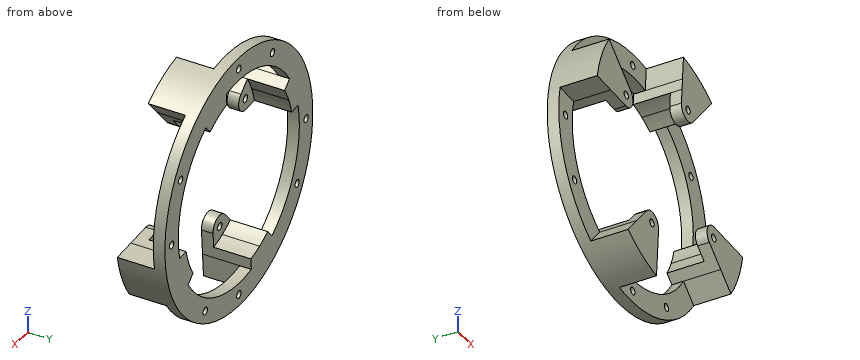
from build123d import *

# Parameters (mm, degrees)
SKETCH1_R           = 55
SKETCH1_R_2         = 1.6
BOSS_EXTRUDE8_DEPTH = 21
CUT_EXTRUDE1_DEPTH  = 16
CUT_EXTRUDE7_START  = 21
SKETCH1_22_R        = 5
SKETCH1_22_R_2      = 1.6
CUT_EXTRUDE7_DEPTH  = 16
SKETCH6_R           = 1.6
CUT_EXTRUDE8_DEPTH  = 81.566742518


with BuildPart() as part:
    # Sketch1 → Boss-Extrude8 (new body)
    with BuildSketch(Plane(origin=(0, 0, 0), x_dir=(1, 0, 0), z_dir=(0, 1, 0))):
        with Locations(Location((0, 0, 0), (0, 0, 90))):
            Circle(SKETCH1_R)
        with BuildLine():
            Line((-24.560877041, 37.706276918), (-17.257446053, 29.262481604))
            ThreePointArc((-17.257446053, 29.262481604), (-11.562365731, 27.91402016), (-8.488842047, 32.894556307))
            Line((-8.488842047, 32.894556307), (-9.295201395, 44.029526809))
            ThreePointArc((-9.295201395, 44.029526809), (17.220754456, 41.574578963), (37.706276918, 24.560877041))
            Line((37.706276918, 24.560877041), (29.262481604, 17.257446053))
            ThreePointArc((29.262481604, 17.257446053), (27.91402016, 11.562365731), (32.894556307, 8.488842047))
            Line((32.894556307, 8.488842047), (44.029526809, 9.295201395))
            ThreePointArc((44.029526809, 9.295201395), (41.574578963, -17.220754456), (24.560877041, -37.706276918))
            Line((24.560877041, -37.706276918), (17.257446053, -29.262481604))
            ThreePointArc((17.257446053, -29.262481604), (11.562365731, -27.91402016), (8.488842047, -32.894556307))
            Line((8.488842047, -32.894556307), (8.94591471, -39.206246783))
            Line((8.94591471, -39.206246783), (9.295201395, -44.029526809))
            ThreePointArc((9.295201395, -44.029526809), (-17.220754456, -41.574578963), (-37.706276918, -24.560877041))
            Line((-37.706276918, -24.560877041), (-34.04871992, -21.39728601))
            Line((-34.04871992, -21.39728601), (-29.262481604, -17.257446053))
            ThreePointArc((-29.262481604, -17.257446053), (-27.91402016, -11.562365731), (-32.894556307, -8.488842047))
            Line((-32.894556307, -8.488842047), (-44.029526809, -9.295201395))
            ThreePointArc((-44.029526809, -9.295201395), (-41.574578963, 17.220754456), (-24.560877041, 37.706276918))
        make_face(mode=Mode.SUBTRACT)
        with Locations(Location((-13.475782892, 32.533417823, 0), (0, 0, 90))):
            Circle(SKETCH1_R_2, mode=Mode.SUBTRACT)
        with Locations(Location((32.533417823, 13.475782892, 0), (0, 0, 90))):
            Circle(SKETCH1_R_2, mode=Mode.SUBTRACT)
        with Locations(Location((-32.533417823, -13.475782892, 0), (0, 0, 90))):
            Circle(SKETCH1_R_2, mode=Mode.SUBTRACT)
        with Locations(Location((13.475782892, -32.533417823, 0), (0, 0, 90))):
            Circle(SKETCH1_R_2, mode=Mode.SUBTRACT)
    extrude(amount=BOSS_EXTRUDE8_DEPTH)

    # Sketch1_15 → Cut-Extrude1 (cut)
    with BuildSketch(Plane(origin=(0, 0, 0), x_dir=(1, 0, 0), z_dir=(0, 1, 0))):
        with BuildLine():
            ThreePointArc((-9.295201395, 44.029526809), (17.220754456, 41.574578963), (37.706276918, 24.560877041))
            Line((37.706276918, 24.560877041), (45.326940374, 31.152343031))
            ThreePointArc((45.326940374, 31.152343031), (21.04758878, 50.813374288), (-10.022953902, 54.079019916))
            Line((-10.022953902, 54.079019916), (-9.295201395, 44.029526809))
        make_face()
        with BuildLine():
            ThreePointArc((-44.029526809, -9.295201395), (-41.574578963, 17.220754456), (-24.560877041, 37.706276918))
            Line((-24.560877041, 37.706276918), (-31.152343031, 45.326940374))
            ThreePointArc((-31.152343031, 45.326940374), (-50.813374288, 21.04758878), (-54.079019916, -10.022953902))
            Line((-54.079019916, -10.022953902), (-44.029526809, -9.295201395))
        make_face()
        with BuildLine():
            Line((54.079019916, 10.022953902), (44.029526809, 9.295201395))
            ThreePointArc((44.029526809, 9.295201395), (41.574578963, -17.220754456), (24.560877041, -37.706276918))
            Line((24.560877041, -37.706276918), (31.152343031, -45.326940374))
            ThreePointArc((31.152343031, -45.326940374), (50.813374288, -21.04758878), (54.079019916, 10.022953902))
        make_face()
        with BuildLine():
            ThreePointArc((9.295201395, -44.029526809), (-17.220754456, -41.574578963), (-37.706276918, -24.560877041))
            Line((-37.706276918, -24.560877041), (-45.326940374, -31.152343031))
            ThreePointArc((-45.326940374, -31.152343031), (-21.04758878, -50.813374288), (10.022953902, -54.079019916))
            Line((10.022953902, -54.079019916), (9.295201395, -44.029526809))
        make_face()
    extrude(amount=CUT_EXTRUDE1_DEPTH, mode=Mode.SUBTRACT)

    # Sketch1_22 → Cut-Extrude7 (cut)
    with BuildSketch(Plane(origin=(0, 0, 0), x_dir=(1, 0, 0), z_dir=(0, 1, 0)).offset(CUT_EXTRUDE7_START)):
        with Locations((13.475782892, -32.533417823)):
            Circle(SKETCH1_22_R)
        with Locations(Location((13.475782892, -32.533417823, 0), (0, 0, 90))):
            Circle(SKETCH1_22_R_2, mode=Mode.SUBTRACT)
        with BuildLine():
            ThreePointArc((15.389200056, -37.152815484), (18.458608875, -35.727285584), (21.39728601, -34.04871992))
            Line((21.39728601, -34.04871992), (17.257446053, -29.262481604))
            ThreePointArc((17.257446053, -29.262481604), (18.16130932, -30.788183712), (18.475782892, -32.533417823))
            ThreePointArc((18.475782892, -32.533417823), (17.633130954, -35.311268987), (15.389200056, -37.152815484))
        make_face()
        with BuildLine():
            ThreePointArc((8.94591471, -39.206246783), (12.210798405, -38.315213416), (15.389200056, -37.152815484))
            ThreePointArc((15.389200056, -37.152815484), (10.849982107, -36.788434889), (8.488842047, -32.894556307))
            Line((8.488842047, -32.894556307), (8.94591471, -39.206246783))
        make_face()
        with BuildLine():
            ThreePointArc((39.206246783, 8.94591471), (38.315213416, 12.210798403), (37.152815486, 15.389200052))
            ThreePointArc((37.152815486, 15.389200052), (37.437344225, 14.451234501), (37.533417823, 13.475782892))
            ThreePointArc((37.533417823, 13.475782892), (36.194407608, 10.070323483), (32.894556307, 8.488842047))
            Line((32.894556307, 8.488842047), (39.206246783, 8.94591471))
        make_face()
        with Locations((32.533417823, 13.475782892)):
            Circle(SKETCH1_22_R)
        with Locations(Location((32.533417823, 13.475782892, 0), (0, 0, 90))):
            Circle(SKETCH1_22_R_2, mode=Mode.SUBTRACT)
        with BuildLine():
            ThreePointArc((37.152815486, 15.389200052), (35.727285585, 18.458608873), (34.04871992, 21.39728601))
            Line((34.04871992, 21.39728601), (29.262481604, 17.257446053))
            ThreePointArc((29.262481604, 17.257446053), (33.685447704, 18.341255855), (37.152815486, 15.389200052))
        make_face()
        with BuildLine():
            Line((-8.488842047, 32.894556307), (-8.94591471, 39.206246783))
            ThreePointArc((-8.94591471, 39.206246783), (-12.210798505, 38.315213384), (-15.38920025, 37.152815404))
            ThreePointArc((-15.38920025, 37.152815404), (-10.849982197, 36.788434944), (-8.488842047, 32.894556307))
        make_face()
        with BuildLine():
            ThreePointArc((-17.257446053, 29.262481604), (-18.34125588, 33.685447599), (-15.38920025, 37.152815404))
            ThreePointArc((-15.38920025, 37.152815404), (-18.458608968, 35.727285536), (-21.39728601, 34.04871992))
            Line((-21.39728601, 34.04871992), (-17.257446053, 29.262481604))
        make_face()
        with Locations((-13.475782892, 32.533417823)):
            Circle(SKETCH1_22_R)
        with Locations(Location((-13.475782892, 32.533417823, 0), (0, 0, 90))):
            Circle(SKETCH1_22_R_2, mode=Mode.SUBTRACT)
        with Locations((-32.533417823, -13.475782892)):
            Circle(SKETCH1_22_R)
        with Locations(Location((-32.533417823, -13.475782892, 0), (0, 0, 90))):
            Circle(SKETCH1_22_R_2, mode=Mode.SUBTRACT)
        with BuildLine():
            ThreePointArc((-29.262481604, -17.257446053), (-33.685447701, -18.341255856), (-37.152815484, -15.389200057))
            ThreePointArc((-37.152815484, -15.389200057), (-35.727285584, -18.458608875), (-34.04871992, -21.39728601))
            Line((-34.04871992, -21.39728601), (-29.262481604, -17.257446053))
        make_face()
        with BuildLine():
            Line((-32.894556307, -8.488842047), (-39.206246783, -8.94591471))
            ThreePointArc((-39.206246783, -8.94591471), (-38.315213416, -12.210798405), (-37.152815484, -15.389200057))
            ThreePointArc((-37.152815484, -15.389200057), (-36.788434889, -10.849982108), (-32.894556307, -8.488842047))
        make_face()
    extrude(amount=-CUT_EXTRUDE7_DEPTH, mode=Mode.SUBTRACT)

    # Sketch6 → Cut-Extrude8 (cut, through all)
    with BuildSketch(Plane(origin=(0, 21, 0), x_dir=(1, 0, 0), z_dir=(0, 1, 0))):
        with Locations(Location((0, 50, 0), (0, 0, 270))):
            Circle(SKETCH6_R)
        with Locations(Location((25, 43.301270189, 0), (0, 0, 270))):
            Circle(SKETCH6_R)
        with Locations(Location((50, 0, 0), (0, 0, 270))):
            Circle(SKETCH6_R)
        with Locations(Location((43.301270189, -25, 0), (0, 0, 270))):
            Circle(SKETCH6_R)
        with Locations(Location((0, -50, 0), (0, 0, 270))):
            Circle(SKETCH6_R)
        with Locations(Location((-25, -43.301270189, 0), (0, 0, 270))):
            Circle(SKETCH6_R)
        with Locations(Location((-50, 0, 0), (0, 0, 270))):
            Circle(SKETCH6_R)
        with Locations(Location((-43.301270189, 25, 0), (0, 0, 270))):
            Circle(SKETCH6_R)
    extrude(amount=-CUT_EXTRUDE8_DEPTH, mode=Mode.SUBTRACT)


solid = part.part
Verification items for the finished model (mm, model axes). Give positions to 0.01 mm unless a question says otherwise; leave off trailing zeros. Write each loop counter-clockwise with the first axis right and the second up, starting at its lowest first coordinate (ties: lowest second). Pieces come first, ordered by that corner, then holes. Notation, with made-up numbers: (43.5, -4) - (61.5, -4) arc R10 cw to (61.5, 5) - close; hole circle Ø10 at (-21.5, 4). An arc over 180 degrees is marked (long way). Answer as CSV lines item,"result". Start each with the question number.
1. Sectioned sample at C-C (z = -6). Record the boundary of the cut face in (x, y).
2. Depth check by flat-ended pin: pin 1 (4 mm diameter, centred on x = -32.53, z = 13.48, fed in from +Y); pin 2 (1.5 mm diameter, centred on y = 14, z = -36, fed in from +X); pin 3 (6 mm diameter, centred on x = -41, y = 13.5, fed in from -Z). Enter the tip coordinate at first touch or a pass-through.
3. Sectioned sample at D-D (x = 50). Record the boundary of the cut face in (y, z), then the cut area to 3 significant figures.
4. Thickness scan on line 1 (X direction, y = 19.8, z = 0); line 2 (X direction, y = 19.9, z = -25); line 3 (Y direction, x = 37, z = 29). Record the ranges inside material, lowest first.
5. Sectioned sample at A-A (y = 12.25). Record the boundary of the cut face in (x, z).
6. Sectioned sample at B-B (x = 0). Record the boundary of the cut face in (y, z), then the cut area to 3 significant figures.
Derived:
1,outline,"(-54.67, 16) - (-44.6, 16) - (-44.6, 21) - (-54.67, 21) - close; (44.6, 16) - (54.67, 16) - (54.67, 21) - (44.6, 21) - close"
2,pin 1,"y = 5"
2,pin 2,"x = -16.33"
2,pin 3,"z = -38.43"
3,outline,"(0, -22.91) - (21, -22.91) - (21, -1.6) - (16, -1.6) - (16, -9.73) - (0, -9.73) - close; (16, 1.6) - (21, 1.6) - (21, 22.91) - (16, 22.91) - close"
3,area,"424 mm²"
4,line 1,"-55 to -51.6, -48.4 to -45, 45 to 48.4, 51.6 to 55"
4,line 2,"-48.99 to -44.9, -41.7 to -37.42, 37.42 to 48.99"
4,line 3,"16 to 21"
5,outline,"(-54.08, 10.02) - (-39.21, 8.95) arc R40.21 cw to (-34.05, 21.4) - (-45.33, 31.15) arc R55 ccw to start; (-31.15, -45.33) arc R55 ccw to (-10.02, -54.08) - (-8.95, -39.21) arc R40.21 cw to (-21.4, -34.05) - close; (8.95, 39.21) arc R40.21 cw to (21.4, 34.05) - (31.15, 45.33) arc R55 ccw to (10.02, 54.08) - close; (34.05, -21.4) - (45.33, -31.15) arc R55 ccw to (54.08, -10.02) - (39.21, -8.95) arc R40.21 cw to start"
6,outline,"(16, -55) - (21, -55) - (21, -51.6) - (16, -51.6) - close; (16, -48.4) - (21, -48.4) - (21, -45) - (16, -45) - close; (16, 45) - (21, 45) - (21, 48.4) - (16, 48.4) - close; (16, 51.6) - (21, 51.6) - (21, 55) - (16, 55) - close"
6,area,"68.0 mm²"
